Study the drawing (mm; zero at the part's minimum x, y, z) and answer. A direction names the side the tool comes from. Give positions to 0.01 mm unless a question says otherwise; leave off trailing zeros. Order: outer loops, then holes, each group sorted by start corner. A loop starts at its lowest first (then second) coordinate and runs counter-clockwise, first axis right, second up.
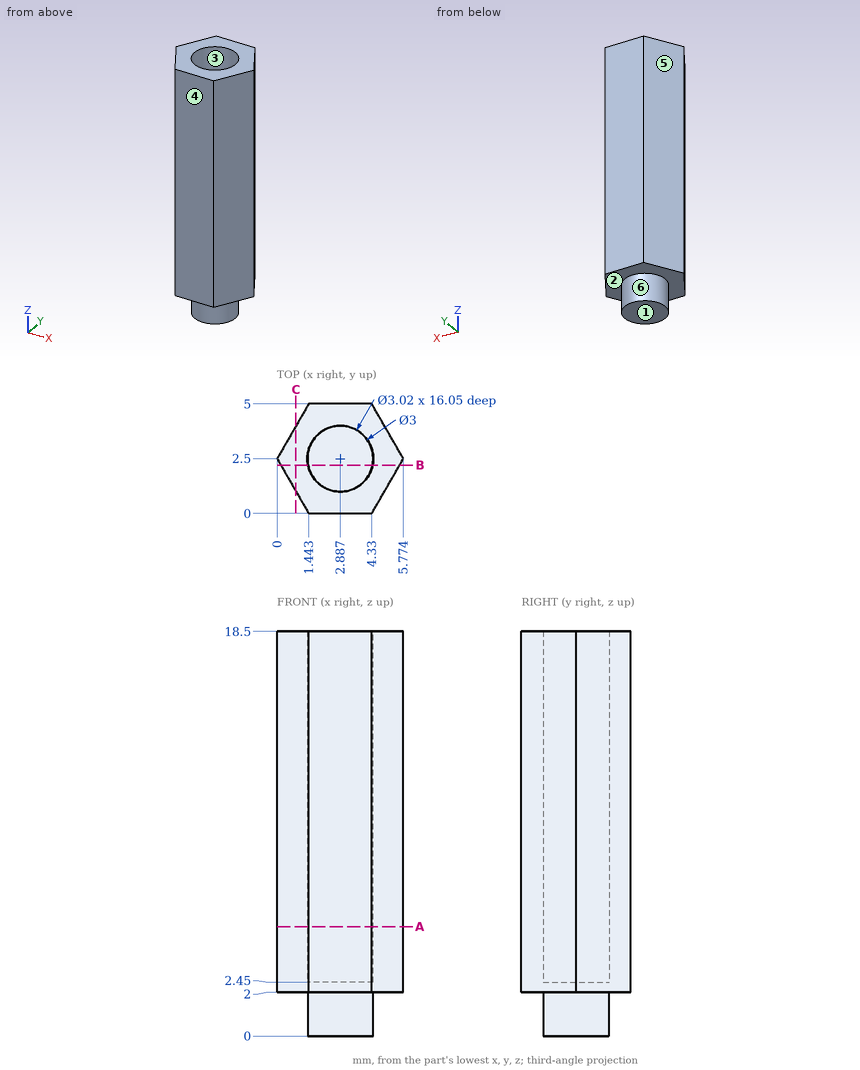
1) A tool of negligible diameter and unlimited length cuts with its end or side. For the marked faces 1 and 2, from which of +Z, -Z, +X, -X, +Y, -Y can it reach the whole face along a straight path? Write none if from no direction.
Geometry says:
face 1: -Z, +X, -X, +Y, -Y
face 2: -Z
2) Given P1, Ø1.5, axis at x = 4.5, y = 0.5, coming from the -Z side, flat-ended and moving along its own axis, determine where the tip first touches the part or whether it passes through.
Geometry says:
P1: stops at z = 2
3) Straight lines are drawn through the part: probe 1 along Y at (x, z) = (2.95, 10.25); probe 2 along X at (y, z) = (2.2, 3.5) (1 decimal); probe 3 along Y at (x, z) = (3.7, 15.25). For each, find the intervals that lie inside material, in ascending order.
Geometry says:
probe 1: y = 0 to 0.99, 4.01 to 5
probe 2: x = 0.2 to 1.4, 4.4 to 5.6
probe 3: y = 0 to 1.23, 3.77 to 5
4) Find section C-C (x = 0.85). Write down the section's boundary in (y, z).
Geometry says:
outline: (1.03, 2) - (3.97, 2) - (3.97, 18.5) - (1.03, 18.5) - close
5) Find section A-A (z = 5). Write down the section's boundary in (x, y).
Geometry says:
outline: (0, 2.5) - (1.44, 0) - (4.33, 0) - (5.77, 2.5) - (4.33, 5) - (1.44, 5) - close; hole circle Ø3.02 at (2.89, 2.5)
6) For a pull along X with two mould halves and no side action, classify the marked faces 3, 4, 5 and 6 as +X half, -X half, draft (parallel to the pull), parting line (faces both ways), or undercut.
Geometry says:
face 3: undercut
face 4: draft
face 5: -X half
face 6: parting line
7) Find section B-B (y = 2.2). Write down the section's boundary in (x, z).
Geometry says:
outline: (0.17, 2) - (1.42, 2) - (1.42, 0) - (4.36, 0) - (4.36, 2) - (5.6, 2) - (5.6, 18.5) - (4.37, 18.5) - (4.37, 2.45) - (1.41, 2.45) - (1.41, 18.5) - (0.17, 18.5) - close
